Part model, mm, in its own coordinate system. A direction names the side the tool comes from. Coordinates: 2 decimals unless noted, no trailing zeros. Loops run counter-clockwise (first coordinate to the right, second up) from the corner with the lowest first, then second, coordinate; pieces in that order, holes last. Notation, with made-up numbers: (-26.75, 83.5) - (-1.75, 83.5) arc R34 ccw to (-1.75, 117.5) - close; hole circle Ø7 at (4, 58.25). An arc over 180 degrees is marked (long way). Use a Markdown table: item, result. Add a question column.
1) Probe probe 1 along Z at (x, y) = (-20, 0); probe 2 along Z at (x, y) = (-5.5, 8.5); probe 3 along Y at (x, z) = (4, 18). List the from-to ranges inside material, lowest first. Write a range as [from, to].
2) Band-saw the part on C-C (x = -30). Give the cut face in (y, z).
3) Pull direction Y, two halves, no side cores. Call faces 1 (the face through (-21.416, -24.672, 139.522)), 2 (the face through (-2.963, -0.871, 29.164)), 3 (the face through (4, -5, 152.4)): +Y half, -Y half, draft (parallel to the pull), parting line (faces both ways), or undercut.
4) Drop a flat-ended pin along its axis: P1, Ø15.5, axis at y = 0, z = 22.53, coming from the -X side. Give the stop position or say it passes through.
5) Band-saw the part on D-D (y = -2.5). Give the cut face in (x, z) (3 decimals), plus the area to 3 significant figures.
6) Band-saw the part on A-A (y = 4.5). Give the cut face in (x, z) (3 decimals).
7) Band-saw the part on B-B (z = 27.5). Give the cut face in (x, y) (3 decimals).
8) Tool access for faces 4 (the face through (-0.265, -8, 139.522)), 5 (the face through (-4, 27.838, 63)): list every direction of +Z, -Z, +X, -X, +Y, -Y with a clear straight run to the whole face (end or side of a thin tool).
from build123d import *

# Parameters (mm, degrees)
F0_W     = 63.97113
F0_H     = 56.596935
F1_DEPTH = 127
F2_R     = 5.418349
F3_DEPTH = 25.4
F4_R     = 6.69388
F5_DEPTH = 85.09
F6_R     = 7.430381
F7_DEPTH = 25.4


with BuildPart() as f1:
    # F0 (on Top) → F1 (new body)
    with BuildSketch(Plane.XY):
        with Locations((-3.410564, -0.460888)):
            Rectangle(F0_W, F0_H)
    extrude(amount=F1_DEPTH)

    # F2 (on face) → F3 (join)
    with BuildSketch(Plane.XY.offset(127)):
        with Locations((4.034519, -4.703406)):
            Circle(F2_R)
    extrude(amount=F3_DEPTH)

    # F4 (on face) → F5 (cut)
    with BuildSketch(Plane.YZ.offset(28.575001)):
        with Locations((0, 22.527253)):
            Circle(F4_R)
    extrude(amount=-F5_DEPTH, mode=Mode.SUBTRACT)

    # F6 (on face) → F7 (join)
    with BuildSketch(Plane.XY.offset(127)):
        with Locations((-24.845107, -18.07957)):
            Circle(F6_R)
    extrude(amount=F7_DEPTH)


solid = f1.part
Answer block:
| question | item | result |
|---|---|---|
| 1 | probe 1 | [0, 15.83], [29.22, 127] |
| 1 | probe 2 | [0, 127] |
| 1 | probe 3 | [-28.76, -4.93], [4.93, 27.84] |
| 2 | outline | (-28.76, 0) - (27.84, 0) - (27.84, 127) - (-12.73, 127) - (-12.73, 152.4) - (-23.43, 152.4) - (-23.43, 127) - (-28.76, 127) - close; hole circle Ø13.39 at (0, 22.53) |
| 3 | face 1 | parting line |
| 3 | face 2 | undercut |
| 3 | face 3 | draft |
| 4 | P1 | x = -35.4 |
| 5 | outline | (-35.396, 0) - (28.575, 0) - (28.575, 16.318) - (-35.396, 16.318) - close; (-35.396, 28.737) - (28.575, 28.737) - (28.575, 127) - (8.985, 127) - (8.985, 152.4) - (-0.916, 152.4) - (-0.916, 127) - (-35.396, 127) - close |
| 5 | area | 7,580 mm2 |
| 6 | outline | (-35.396, 0) - (28.575, 0) - (28.575, 17.572) - (-35.396, 17.572) - close; (-35.396, 27.483) - (28.575, 27.483) - (28.575, 127) - (-35.396, 127) - close |
| 7 | outline | (-35.396, -28.759) - (28.575, -28.759) - (28.575, -4.481) - (-35.396, -4.481) - close; (-35.396, 4.481) - (28.575, 4.481) - (28.575, 27.838) - (-35.396, 27.838) - close |
| 8 | face 4 | +Z |
| 8 | face 5 | +Z, -Z, +X, -X, +Y |
